from build123d import *

# Parameters (mm, degrees)
F0_W           = 147.32
F0_H           = 71.12
F1_DEPTH       = 38.1
F3_DEPTH       = 76.201
F4_R           = 10.16
F5_DEPTH       = 76.201
F6_W           = 10.16
F6_H           = 76.2
F7_DEPTH       = 10.16
F8_D           = 15.24
F8_CBORE_D     = 40.64
F8_CBORE_DEPTH = 10.16
F10_DEPTH      = 27.94


with BuildPart() as f1:
    # F0 (on Right) → F1 (new body, symmetric)
    with BuildSketch(Plane.YZ):
        with Locations((0, 35.56)):
            Rectangle(F0_W, F0_H)
    extrude(amount=F1_DEPTH, both=True)

    # F2 (on face) → F3 (cut, through all)
    with BuildSketch(Plane.YZ.offset(38.1)):
        Polygon((2.54, 35.56), (38.1, 71.12), (-73.66, 71.12), (-73.66, 35.56), align=None)
        Polygon((73.66, 35.56), (38.1, 0), (73.66, 0), align=None)
    extrude(amount=-F3_DEPTH, mode=Mode.SUBTRACT)

    # F4 (on face) → F5 (cut, through all)
    with BuildSketch(Plane.YZ.offset(38.1)):
        with Locations((20.32, 20.32)):
            Circle(F4_R)
    extrude(amount=-F5_DEPTH, mode=Mode.SUBTRACT)

    # F6 (on face) → F7 (cut)
    with BuildSketch(Plane.XY.offset(35.56)):
        with Locations((0, -35.56)):
            Rectangle(F6_W, F6_H)
    extrude(amount=-F7_DEPTH, mode=Mode.SUBTRACT)

    # F8 (through all)
    with Locations(Plane.XY.offset(35.56)):
        with Locations((0, -35.56)):
            CounterBoreHole(F8_D / 2, F8_CBORE_D / 2, F8_CBORE_DEPTH)

    # F9 (on face) → F10 (cut)
    with BuildSketch(Plane.XY.offset(71.12)):
        with BuildLine():
            Line((22.86, 59.69), (-22.86, 59.69))
            ThreePointArc((-22.86, 59.69), (-26.67, 55.88), (-22.86, 52.07))
            Line((-22.86, 52.07), (22.86, 52.07))
            ThreePointArc((22.86, 52.07), (26.67, 55.88), (22.86, 59.69))
        make_face()
    extrude(amount=-F10_DEPTH, mode=Mode.SUBTRACT)


solid = f1.part
Design review of the part built by this model. Coordinates are the model's own, in mm. A direction names the side the tool comes from. Coordinates: 2 decimals unless noted, no trailing zeros. Loops run counter-clockwise (first coordinate to the right, second up) from the corner with the lowest first, then second, coordinate; pieces in that order, holes last. Notation, with made-up numbers: (13.25, 31) -> (66.25, 31) arc R14 ccw to (66.25, 41) -> close; hole circle Ø2 at (-39, 16.25). An arc over 180 degrees is marked (long way). Use a Markdown table: item, result. Add a question column.
Item 1: We need section D-D, the plane x = 30.5. Write out the cut boundary in (y, z), and give its area (3 significant figures).
Item 2: We need section A-A, the plane z = 20.32. Write out the cut boundary in (x, y).
Item 3: Machinability: for faces 1 (the flat face through (-25, -36, 35.56)), 2 (the flat face through (0, 2.54, 31)), 3 (the cylindrical face through (26.67, 55.8, 57.35)), which of the approach directions +Z, -Z, +X, -X, +Y, -Y give a long, thin tool a straight path to every point of the face, cutting with its end or side? Answer none if there is none.
Item 4: We need section C-C, the plane x = 0. Write out the cut boundary in (y, z).
Item 5: We need section B-B, the plane y = -35.56. Write out the cut boundary in (x, z).
Item 6: The part is to be moulded in two halves that separate along Y. For faces 4 (the flat face through (-5.08, -7, 31)), 5 (the cylindrical face through (20.317, -35.935, 30.551)), 6 (the flat face through (1, 73.66, 53)), say which applies: +Y half, -Y half, draft (parallel to the pull), parting line (faces both ways), or undercut.
Item 7: Wall thickness on L1, parallel to Y at x = 0, z = 12; L2, parallel to Z at x = -2, y = -26; L3, parallel to Y at x = -24.5, z = 20: over which ranges is each line inside the solid? List them lowest first. Write a range as from..to.
Item 8: Clearance check with flat-ended pins moving along their axes: P1, Ø12, axis at x = 30.5, z = 43.5, coming from the -Y side; P2, Ø10, axis at x = -12, y = -25, coming from the +Z side; P3, Ø4, axis at x = 28.5, y = 26, coming from the +Z side; P4, Ø23.5, axis at y = 20.32, z = 20.32, coming from the +X side. State where each tip first meets the part, or that it passes through.
Numbers:
| question | item | result |
|---|---|---|
| 1 | outline | (-73.66, 0) -> (38.1, 0) -> (73.66, 35.56) -> (73.66, 71.12) -> (38.1, 71.12) -> (2.54, 35.56) -> (-73.66, 35.56) -> close; hole circle Ø20.32 at (20.32, 20.32) |
| 1 | area | 6,180 mm^2 |
| 2 | outline | (-38.1, -73.66) -> (38.1, -73.66) -> (38.1, 10.16) -> (-38.1, 10.16) -> close; (-38.1, 30.48) -> (38.1, 30.48) -> (38.1, 58.42) -> (-38.1, 58.42) -> close; hole circle Ø15.24 at (0, -35.56) |
| 3 | face 1 | +Z, +X, -X, -Y |
| 3 | face 2 | +Z, -Y |
| 3 | face 3 | +Z |
| 4 | outline | (-73.66, 0) -> (-43.18, 0) -> (-43.18, 25.4) -> (-73.66, 25.4) -> close; (-27.94, 0) -> (38.1, 0) -> (73.66, 35.56) -> (73.66, 71.12) -> (59.69, 71.12) -> (59.69, 43.18) -> (52.07, 43.18) -> (52.07, 71.12) -> (38.1, 71.12) -> (2.54, 35.56) -> (2.54, 25.4) -> (-27.94, 25.4) -> close; hole circle Ø20.32 at (20.32, 20.32) |
| 5 | outline | (-38.1, 0) -> (-7.62, 0) -> (-7.62, 25.4) -> (-20.32, 25.4) -> (-20.32, 35.56) -> (-38.1, 35.56) -> close; (7.62, 0) -> (38.1, 0) -> (38.1, 35.56) -> (20.32, 35.56) -> (20.32, 25.4) -> (7.62, 25.4) -> close |
| 6 | face 4 | draft |
| 6 | face 5 | undercut |
| 6 | face 6 | +Y half |
| 7 | L1 | y = -73.66..-43.18, -27.94..14.49, 26.15..50.1 |
| 7 | L2 | z = 0..25.4 |
| 7 | L3 | y = -73.66..10.17, 30.47..58.1 |
| 8 | P1 | stops at y = 4.48 |
| 8 | P2 | stops at z = 35.56 |
| 8 | P3 | stops at z = 61.02 |
| 8 | P4 | stops at x = 38.1 |
